Work out the finished part from the listing and answer in its coordinate system (mm). Round coordinates to 2 decimals unless told otherwise and drop trailing zeros. Write each loop counter-clockwise with the first axis right and the second up, starting at its lowest first coordinate (ties: lowest second). Pieces come first, ordered by that corner, then holes.
1. Determine the mould class of faces 1 (the face through (6.35, 56, 13)), 2 (the face through (3, 58, 25.4)), 3 (the face through (3.131, 82.556, 12.421)) for opening direction Z: pulls with the +Z half, pulls with the -Z half, needs draft (parallel to the pull), parting line crosses it, or undercut.
2. Find section B-B (z = 12.7). Write down the section's boundary in (x, y).
3. Find section C-C (x = 3.25). Write down the section's boundary in (y, z).
4. Find section D-D (y = 22). Write down the section's boundary in (x, z), and give its area (3 significant figures).
5. Find section A-A (y = 88.9). Write down the section's boundary in (x, z).
6. Straight lines are drawn through the part: probe 1 along Z at (x, y) = (5, 88.9); probe 2 along Y at (x, z) = (2, 10.5); probe 3 along Y at (x, z) = (3.5, 16.25). For each, find the intervals that lie inside material, in ascending order.
Autodesk Inventor part; units mm, degrees
ref_plane "YZ Plane" through (0, 0, 0) normal (1, 0, 0) x (0, 1, 0)
ref_plane "XZ Plane" through (0, 0, 0) normal (0, 1, 0) x (-1, 0, 0)
ref_plane "XY Plane" through (0, 0, 0) normal (0, 0, 1) x (1, 0, 0)
sketch "Sketch1" plane through (0, 0, 0) normal (1, 0, 0) x (0, 1, 0)
  line L0 (0, 0) -> (114.3, 0)
  line L1 (114.3, 0) -> (114.3, 25.4)
  line L2 (114.3, 25.4) -> (0, 25.4)
  line L3 (0, 25.4) -> (0, 0)
  line L4 (114.3, 12.7) -> (88.9, 12.7)
  line L5 (88.9, 12.7) -> (25.4, 12.7)
  circle A0 centre (25.4, 12.7) radius 6.35
  circle A1 centre (88.9, 12.7) radius 6.35
  dimension "d0" = 114.3
  dimension "d1" = 25.4
  dimension "d4" = 25.4
  dimension "d5" = 63.5
  dimension "d6" = 12.7
  dimension "d7" = 12.7
extrude "Extrusion2" add sketch "Sketch1" along normal blind 6.35
properties part number "CatapultArmSquare-Thickener"
Worked answers:
1. face 1: needs draft
1. face 2: pulls with the +Z half
1. face 3: undercut
2. outline: (0, 0) - (6.35, 0) - (6.35, 19.05) - (0, 19.05) - close; (0, 31.75) - (6.35, 31.75) - (6.35, 82.55) - (0, 82.55) - close; (0, 95.25) - (6.35, 95.25) - (6.35, 114.3) - (0, 114.3) - close
3. outline: (0, 0) - (114.3, 0) - (114.3, 25.4) - (0, 25.4) - close; hole circle Ø12.7 at (25.4, 12.7); hole circle Ø12.7 at (88.9, 12.7)
4. outline: (0, 0) - (6.35, 0) - (6.35, 7.34) - (0, 7.34) - close; (0, 18.06) - (6.35, 18.06) - (6.35, 25.4) - (0, 25.4) - close
4. area: 93.2 mm2
5. outline: (0, 0) - (6.35, 0) - (6.35, 6.35) - (0, 6.35) - close; (0, 19.05) - (6.35, 19.05) - (6.35, 25.4) - (0, 25.4) - close
6. probe 1: z = 0 to 6.35, 19.05 to 25.4
6. probe 2: y = 0 to 19.44, 31.36 to 82.94, 94.86 to 114.3
6. probe 3: y = 0 to 20.14, 30.66 to 83.64, 94.16 to 114.3
